Build history of the part. All positions in model axes, mm. Face numbers are marked on the shaded views. Give positions to 0.01 mm unless a question says otherwise; leave off trailing zeros. Write each loop counter-clockwise with the first axis right and the second up, starting at its lowest first coordinate (ties: lowest second). Pieces come first, ordered by that corner, then holes. Notation, with made-up numbers: (23.25, 8) -> (50.25, 8) arc R12 cw to (50.25, 30) -> close; hole circle Ø11 at (85.5, -21.5). An arc over 180 degrees is marked (long way). Put each result on its own line as item: value.
from build123d import *

# Parameters (mm, degrees)
ESQUISSE1_R             = 2.95
ESQUISSE1_R_2           = 1
BOSS_EXTRU_1_DEPTH      = 8
ENL_V_START             = -6
ENL_V_MAT_EXTRU_1_DEPTH = 6


with BuildPart() as part:
    # Esquisse1 → Boss.-Extru.1 (new body)
    with BuildSketch(Plane.XY):
        with BuildLine():
            Line((0, 5), (26.5, 2.5))
            ThreePointArc((26.5, 2.5), (29, 0), (26.5, -2.5))
            Line((26.5, -2.5), (0, -5))
            ThreePointArc((0, -5), (-5, 0), (0, 5))
        make_face()
        Circle(ESQUISSE1_R, mode=Mode.SUBTRACT)
        with Locations((26.5, 0)):
            Circle(ESQUISSE1_R_2, mode=Mode.SUBTRACT)
    extrude(amount=BOSS_EXTRU_1_DEPTH)

    # Esquisse2 → Enlèv. mat.-Extru.1 (cut)
    with BuildSketch(Plane.XY.offset(8).offset(ENL_V_START)):
        with BuildLine():
            Line((26.5, 2.5), (0.9350741, 4.911785462))
            ThreePointArc((0.9350741, 4.911785462), (3.851971606, 3.18783857), (5, 0))
            ThreePointArc((5, 0), (3.851971606, -3.18783857), (0.9350741, -4.911785462))
            Line((0.9350741, -4.911785462), (26.5, -2.5))
            ThreePointArc((26.5, -2.5), (24, 0), (26.5, 2.5))
        make_face()
        with BuildLine():
            ThreePointArc((29, 0), (28.348574488, 1.683084182), (26.73378211, 2.489045183))
            Line((26.73378211, 2.489045183), (26.663377196, 0.986563679))
            ThreePointArc((26.663377196, 0.986563679), (27.262685124, 0.646769976), (27.5, 0))
            ThreePointArc((27.5, 0), (27.231575326, -0.68176062), (26.570404914, -0.997518495))
            Line((26.570404914, -0.997518495), (26.5, -2.5))
            ThreePointArc((26.5, -2.5), (28.267766953, -1.767766953), (29, 0))
        make_face()
        with BuildLine():
            Line((26.663377196, 0.986563679), (26.73378211, 2.489045183))
            ThreePointArc((26.73378211, 2.489045183), (26.617019318, 2.497259794), (26.5, 2.5))
            ThreePointArc((26.5, 2.5), (24, 0), (26.5, -2.5))
            Line((26.5, -2.5), (26.570404914, -0.997518495))
            ThreePointArc((26.570404914, -0.997518495), (25.501096082, 0.046807727), (26.663377196, 0.986563679))
        make_face()
    extrude(amount=ENL_V_MAT_EXTRU_1_DEPTH, mode=Mode.SUBTRACT)


solid = part.part
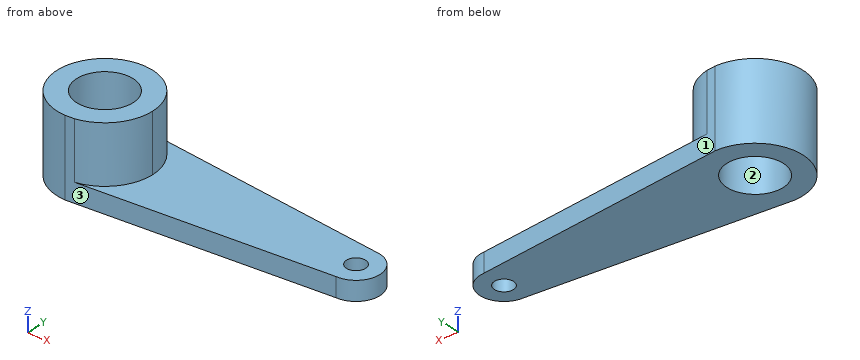
1) Slice it at A-A (x = -1.5). Write the cut outline in (y, z), plus the area to 3 significant figures.
Filled sheet:
outline: (-4.77, 0) -> (-2.54, 0) -> (-2.54, 8) -> (-4.77, 8) -> close; (2.54, 0) -> (4.77, 0) -> (4.77, 8) -> (2.54, 8) -> close
area: 35.7 mm2
2) Wall check: L1, parallel to Y at x = 26.5, z = 1.6; L2, parallel to Z at x = 14, y = -3.25; L3, parallel to Y at x = 2, z = 7.25. Give the ranges that are in metal, low to high.
Filled sheet:
L1: -2.5 to -1, 1 to 2.5
L2: 0 to 2
L3: -4.58 to -2.17, 2.17 to 4.58
3) Pin check, flat tip, straight feed: pin 1 (1 mm diameter, centred on x = 15, z = 3, fed in from -Y). Stop position of the tip, or through.
Filled sheet:
pin 1: through
4) Slice it at B-B (z = 0.5). Write the cut outline in (x, y), plus the area to 3 significant figures.
Filled sheet:
outline: (0, -5) -> (26.5, -2.5) arc R2.5 ccw to (26.5, 2.5) -> (0, 5) arc R5 ccw to start; hole circle Ø5.9 at (0, 0); hole circle Ø2 at (26.5, 0)
area: 217 mm2
5) Slice it at C-C (z = 2.5). Write the cut outline in (x, y).
Filled sheet:
outline: (0, -5) -> (0.94, -4.91) arc R5 ccw to (0.94, 4.91) -> (0, 5) arc R5 ccw to start; hole circle Ø5.9 at (0, 0)
6) Slice it at D-D (x = 4.5). Write the cut outline in (y, z), plus the area to 3 significant figures.
Filled sheet:
outline: (-4.58, 0) -> (4.58, 0) -> (4.58, 2) -> (2.18, 2) -> (2.18, 8) -> (-2.18, 8) -> (-2.18, 2) -> (-4.58, 2) -> close
area: 44.5 mm2
7) Pull direction Y, two halves, no side cores. Call the marked faces 1, 2 and 3: released by +Y, released by -Y, zero draft, split by the parting line, or undercut.
Filled sheet:
face 1: released by +Y
face 2: undercut
face 3: released by -Y
